Autodesk Inventor part; units mm, degrees
ref_plane "YZ Plane" through (0, 0, 0) normal (1, 0, 0) x (0, 1, 0)
ref_plane "XZ Plane" through (0, 0, 0) normal (0, 1, 0) x (-1, 0, 0)
ref_plane "XY Plane" through (0, 0, 0) normal (0, 0, 1) x (1, 0, 0)
sketch "Sketch1" plane through (0, 0, 0) normal (0, 1, 0) x (-1, 0, 0)
  line L0 (101.6, -101.6) -> (-101.6, -101.6)
  line L1 (-101.6, -101.6) -> (-101.6, 101.6)
  line L2 (-101.6, 101.6) -> (101.6, 101.6)
  line L3 (101.6, 101.6) -> (101.6, -101.6)
  line L4 (96.6, -96.6) -> (-96.6, -96.6)
  line L5 (-96.6, -96.6) -> (-96.6, 96.6)
  line L6 (-96.6, 96.6) -> (96.6, 96.6)
  line L7 (96.6, 96.6) -> (96.6, -96.6)
  line L8 (101.6, 101.6) -> (-40.4, 101.6)
  circle A0 centre (0, 0) radius 88.9
  line L9 (-40.4, 101.6) -> (-101.6, 40.4)
  line L10 (-45.4, 101.6) -> (-101.6, 45.4)
  line L11 (96.6, 96.6) -> (96.6, 101.6)
  line L12 (-45.4, 101.6) -> (-35.4, 101.6)
  line L13 (-35.4, 101.6) -> (-35.4, 96.6)
  line L14 (-35.4, 96.6) -> (-45.4, 96.6)
  line L15 (-45.4, 96.6) -> (-45.4, 101.6)
  line L16 (-101.6, 39.4) -> (-39.4, 101.6)
  line L17 (96.4, -96.4) -> (-96.4, -96.4)
  line L18 (-96.4, -96.4) -> (-96.4, 96.4)
  line L19 (-96.4, 96.4) -> (96.4, 96.4)
  line L20 (96.4, 96.4) -> (96.4, -96.4)
  circle A1 centre (0, 0) radius 90.9
  point P0 (96.6, 51.2168)
  point P1 (101.6, 40.4)
  point P2 (101.6, -40.4)
  point P3 (96.6, -51.2168)
  point P4 (-96.6, 45.4)
  point P5 (-45.4, 96.6)
  point P6 (-44.6, 96.4)
  point P7 (-96.4, 44.6)
  dimension "d0" = 203.2
  dimension "d1" = 203.2
  dimension "d2" = 101.6
  dimension "d3" = 101.6
  dimension "d4" = 5
  dimension "d5" = 5
  dimension "d6" = 5
  dimension "d7" = 5
  dimension "d8" = 142
  dimension "d9" = 61.2
  dimension "d10" = 177.8
  dimension "d11" = 5
  dimension "d12" = 5
  dimension "d13" = 10
  dimension "d14" = 1
  dimension "d15" = 0.2
  dimension "d16" = 0.2
  dimension "d17" = 0.2
  dimension "d18" = 0.2
  dimension "d64" = 181.8
extrude "Extrusion1" add sketch "Sketch1" along normal blind 4 contours L16 L19 L20 L17 L18
sketch "Sketch6" plane through (0, 4, 0) normal (0, 1, 0) x (1, 0, 0)
  line L0 (96.4, 96.4) -> (-96.4, 96.4)
  line L1 (96.4, 96.4) -> (88.4, 96.4)
  line L2 (88.4, 96.4) -> (88.4, -45.6)
  line L3 (88.4, -45.6) -> (96.4, -45.6)
  line L4 (96.4, -45.6) -> (96.4, 96.4)
  line L5 (96.4, -44.6) -> (96.4, 96.4)
  line L6 (88.4, -12) -> (96.4, -12)
  line L7 (96.4, -12) -> (96.4, 12)
  line L8 (96.4, 12) -> (88.4, 12)
  line L9 (88.4, 12) -> (88.4, -12)
  line L10 (0, 0) -> (96.4, 0)
  point P0 (96.4, -12)
  dimension "d58" = 8
  dimension "d59" = 142
  dimension "d62" = 12
  dimension "d63" = 12
extrude "Extrusion6" cut sketch "Sketch6" against normal blind 25.4 contours L4 L10 L2 L8 | L4 L6 L2 L10
sketch "Sketch8" plane through (0, 4, 0) normal (0, 1, 0) x (1, 0, 0)
  line L0 (-96.6, 96.6) -> (-96.6, -96.6)
  line L1 (96.6, 96.6) -> (-96.6, 96.6)
  line L2 (-96.6, 96.6) -> (96.6, 96.6)
  line L3 (96.6, -45.4) -> (45.4, -96.6)
  line L4 (96.6, 96.6) -> (96.6, -45.4)
  line L5 (96.6, -45.4) -> (45.4, -96.6)
  line L6 (45.4, -96.6) -> (-96.6, -96.6)
  line L7 (-96.6, -96.6) -> (-96.6, 96.6)
  line L8 (-96.6, 96.6) -> (-89.5289, 89.5289)
  circle A0 centre (-89.5289, 89.5289) radius 5
  circle A1 centre (-89.5289, 89.5289) radius 1.5
  line L9 (-89.5289, 84.5289) -> (-96.6, 84.5289)
  line L10 (-89.5289, 89.5289) -> (-89.5289, 84.5289)
  line L11 (-89.5289, 89.5289) -> (-84.5289, 89.5289)
  line L12 (-84.5289, 96.6) -> (-84.5289, 89.5289)
  line L13 (-96.6, -96.6) -> (-89.5289, -89.5289)
  line L14 (-96.6, -96.6) -> (-86.6, -96.6) construction
  circle A2 centre (-89.5289, -89.5289) radius 5
  circle A3 centre (-89.5289, -89.5289) radius 1.75
  line L15 (-89.5289, -89.5289) -> (-84.5289, -89.5289)
  line L16 (-84.5289, -96.6) -> (-84.5289, -89.5289)
  line L17 (-89.5289, -89.5289) -> (-89.5289, -84.5289)
  line L18 (-96.6, -84.5289) -> (-89.5289, -84.5289)
  line L19 (96.6, 96.6) -> (89.5289, 89.5289)
  circle A4 centre (89.5289, 89.5289) radius 5
  circle A5 centre (89.5289, 89.5289) radius 1.75
  line L20 (89.5289, 89.5289) -> (84.5289, 89.5289)
  line L21 (84.5289, 96.6) -> (84.5289, 89.5289)
  line L22 (89.5289, 89.5289) -> (89.5289, 84.5289)
  line L23 (96.6, 84.5289) -> (89.5289, 84.5289)
  line L24 (96.6, -43.114) -> (96.6, 96.6)
  line L25 (-96.6, -96.6) -> (43.1178, -96.6)
  line L26 (28.9914, 5.6569) -> (-5.6569, -28.9914)
  line L27 (25.4, -25.4) -> (101.6, -25.4)
  line L28 (101.6, -88.9) -> (101.6, 101.6)
  line L29 (25.4, -25.4) -> (25.4, -101.6)
  line L30 (43.1178, -101.6) -> (-101.6, -101.6)
  line L31 (96.6, -25.4) -> (86.6, -25.4)
  circle A6 centre (86.6, -25.4) radius 5
  circle A7 centre (86.6, -25.4) radius 1.75
  line L32 (25.4, -96.6) -> (25.4, -86.6)
  circle A8 centre (25.4, -86.6) radius 5
  circle A9 centre (25.4, -86.6) radius 1.75
  line L33 (44.6, -96.4) -> (96.4, -44.6)
  circle A10 centre (68.7322, -68.7322) radius 1
  point P0 (0, 0)
  point P1 (0, 0)
  point P2 (0, 0)
  dimension "d90" = 10
  dimension "d91" = 3
  dimension "d92" = 10
  dimension "d93" = 45
  dimension "d94" = 10
  dimension "d95" = 3.5
  dimension "d96" = 10
  dimension "d97" = 10
  dimension "d98" = 3.5
  dimension "d99" = 76.2
  dimension "d100" = 76.2
  dimension "d101" = 10
  dimension "d102" = 10
  dimension "d103" = 3.5
  dimension "d104" = 10
  dimension "d105" = 10
  dimension "d106" = 3.5
  dimension "d115" = 2
  dimension "d116" = 2.5
hole "Hole1" at (-89.5289, 4, -89.5289) at (89.5289, 4, -89.5289) at (-89.5289, 4, 89.5289) at (68.7322, 4, 68.7322) direction (0, -1, 0) diameter 3.1211 depth 2.75 tip angle 118 countersink diameter 3.2004 countersink angle 82
fillet "Fillet1" radius 3.175 2 edges at (-6.0132, 0, -90.7009) (-6.0132, 0, 90.7009)
sketch "Sketch9" plane through (0, 4, 0) normal (0, 1, 0) x (1, 0, 0)
  arc A0 (-101.6, -98.425) -> (-98.425, -101.6) centre (-98.425, -98.425) ccw
  line L0 (44.0849, 101.6) -> (-98.425, 101.6)
  line L1 (-101.6, 98.425) -> (-101.6, -98.425)
  line L2 (-101.6, -46.1) -> (-101.6, -76.6)
  line L3 (-96.6, -96.6) -> (-96.6, 96.6)
  line L4 (-96.6, -46.1) -> (-96.6, -76.6)
  line L5 (-101.6, -76.6) -> (-96.6, -76.6)
  line L6 (-101.6, -46.1) -> (-96.6, -46.1)
  line L7 (-98.425, -101.6) -> (101.6, -101.6)
  line L8 (0, 0) -> (-101.6, 0)
  line L9 (-101.6, 46.1) -> (-101.6, 76.6)
  line L10 (-96.6, 46.1) -> (-96.6, 76.6)
  line L11 (-101.6, 76.6) -> (-96.6, 76.6)
  line L12 (-101.6, 46.1) -> (-96.6, 46.1)
  line L13 (-96.6, -76.6) -> (-90.1, -76.6)
  line L14 (-90.1, -76.6) -> (-90.1, -46.1)
  line L15 (-90.1, -46.1) -> (-96.6, -46.1)
  line L16 (-96.6, -46.1) -> (-96.6, -76.6)
  arc A1 (-98.425, 101.6) -> (-101.6, 98.425) centre (-98.425, 98.425) ccw
  line L17 (-101.6, 46.1) -> (-96.6, 46.1)
  line L18 (-90.1, 46.1) -> (-96.6, 46.1)
  line L19 (-101.6, 46.1) -> (-101.6, 76.6)
  line L20 (-96.6, 46.1) -> (-96.6, 76.6)
  line L21 (-96.6, 46.1) -> (-96.6, 76.6)
  line L22 (-90.1, 76.6) -> (-90.1, 46.1)
  line L23 (-101.6, 76.6) -> (-96.6, 76.6)
  line L24 (-96.6, 76.6) -> (-90.1, 76.6)
  point P0 (-98.425, 98.425)
  point P1 (46.1, 101.6)
  point P2 (46.1, 96.6)
  point P3 (76.6, 96.6)
  point P4 (76.6, 101.6)
  point P5 (-46.1, 96.6)
  dimension "d117" = 30.5
  dimension "d118" = 25
  dimension "d119" = 6.5
extrude "Extrusion7" cut sketch "Sketch9" against normal blind 25.4 contours L24 L22 L18 L3 | L15 L14 L13 L3
sketch "Sketch10" plane through (0, 4, 0) normal (0, 1, 0) x (1, 0, 0)
  line L0 (-96.3514, 0) -> (-90.9, 0)
  arc A0 (90.1044, 12) -> (90.1044, -12) centre (0, 0) ccw
ref_plane "Work Plane1" through (-96.3514, 4, 0) normal (0, 0, 1) x (1, 0, 0)
sketch "Sketch11" plane through (-96.3514, 4, 0) normal (0, 0, 1) x (1, 0, 0)
  line L0 (-51.1439, 37.1405) -> (237.6314, 37.1405)
  line L1 (237.6314, 37.1405) -> (237.6314, -59.6996)
  line L2 (237.6314, -59.6996) -> (-51.1439, -59.6996)
  line L3 (-51.1439, -59.6996) -> (-51.1439, 37.1405)
  point P0 (96.3514, -4)
extrude "Extrusion8" cut sketch "Sketch11" along normal through all
equation "\"d1\" = d0"
equation "\"d15\" = d17"
equation "\"d16\" = d17"
equation "\"d18\" = d17"
properties part number "Drop_Plate"
Check sheet for the modelled part. Datum: model origin and axes. Units: mm. A direction names the side the tool comes from. Round coordinates to 2 decimals unless told otherwise and drop trailing zeros. Order: outer loops, then holes, each group sorted by start corner. A loop starts at its lowest first (then second) coordinate and runs counter-clockwise, first axis right, second up.
Q1. Scan lines: L1, parallel to X at y = 3.2, z = -27; L2, parallel to X at y = 2.9, z = -32.5; L3, parallel to X at y = 1.95, z = -7. Record each from-to range of solid material in increasing order.
Filled sheet:
L1: x = -96.4 to -86.8, 86.8 to 96.4
L2: x = -96.4 to -84.9, 84.9 to 96.4
L3: x = -96.4 to -90.88
Q2. Cross-section at B-B, the plane x = 0. Enter the section's corners in (y, z) (3 decimals), plus the area to 3 significant figures.
Filled sheet:
outline: (0, -96.4) - (4, -96.4) - (4, -90.9) - (3.175, -90.9) arc R3.175 ccw to (0, -94.075) - close
area: 19.8 mm2
Q3. Set-up check for faces 1 (the face through (8, 4, -94)), 2 (the face through (93, 2, -12)), 3 (the face through (-90.1, 2, -62)): record each of +Z, -Z, +X, -X, +Y, -Y from which the full face is reachable in a straight line by a thin tool's end or side.
Filled sheet:
face 1: +Z, -Z, +X, -X, +Y
face 2: +Z, +X, +Y, -Y
face 3: -X, +Y, -Y
Q4. Cross-section at A-A, the plane y = 2.45. Enter the section's corners in (x, z), plus the area to 3 significant figures.
Filled sheet:
outline: (-96.4, -96.4) - (96.4, -96.4) - (96.4, -12) - (90.19, -12) arc R90.98 cw to (-90.98, 0) - (-96.4, 0) - (-96.4, -46.1) - (-90.1, -46.1) - (-90.1, -76.6) - (-96.4, -76.6) - close; hole circle Ø3.12 at (-89.53, -89.53); hole circle Ø3.12 at (89.53, -89.53)
area: 5,310 mm2
Q5. Depth check by flat-ended pin: P1, Ø1, axis at x = -69, y = 2.5, coming from the +Z side; P2, Ø2, axis at y = 1, z = -62, coming from the -X side; P3, Ø1.2, axis at x = 94.5, y = 2, coming from the +Z side. Enter the tip coordinate at first touch or a pass-through.
Filled sheet:
P1: stops at z = -58.68
P2: stops at x = -90.1
P3: stops at z = -12
Q6. Draft check along X on faces 4 (the face through (-96.4, 2, -86)), 5 (the face through (-94, 2, 0)), 6 (the face through (-7.922, 3.582, -90.554)), 7 (the face through (96.4, 2, -55)). Enter one of: pulls with the +X half, pulls with the -X half, needs draft (parallel to the pull), parting line crosses it, or undercut.
Filled sheet:
face 4: pulls with the -X half
face 5: needs draft
face 6: undercut
face 7: pulls with the +X half
